```python
from build123d import *

# Parameters (mm, degrees)
SKETCH1_R           = 55
SKETCH1_R_2         = 3
BOSS_EXTRUDE1_DEPTH = 10
CUT_EXTRUDE1_DEPTH  = 10


with BuildPart() as part:
    # Sketch1 → Boss-Extrude1 (new body)
    with BuildSketch(Plane.XY):
        Circle(SKETCH1_R)
        Circle(SKETCH1_R_2, mode=Mode.SUBTRACT)
    extrude(amount=BOSS_EXTRUDE1_DEPTH)

    # Sketch2 → Cut-Extrude1 (cut)
    with BuildSketch(Plane.XY.offset(10)):
        with BuildLine():
            Line((-50.754310162, -5), (-46.733285782, -5))
            ThreePointArc((-46.733285782, -5), (0, -47), (46.733285782, -5))
            Line((46.733285782, -5), (50.754310162, -5))
            ThreePointArc((50.754310162, -5), (0, -51), (-50.754310162, -5))
        make_face()
        with BuildLine():
            Line((-50.754310162, 5), (-46.733285782, 5))
            ThreePointArc((-46.733285782, 5), (0, 47), (46.733285782, 5))
            Line((46.733285782, 5), (50.754310162, 5))
            ThreePointArc((50.754310162, 5), (0, 51), (-50.754310162, 5))
        make_face()
    extrude(amount=-CUT_EXTRUDE1_DEPTH, mode=Mode.SUBTRACT)


solid = part.part
```
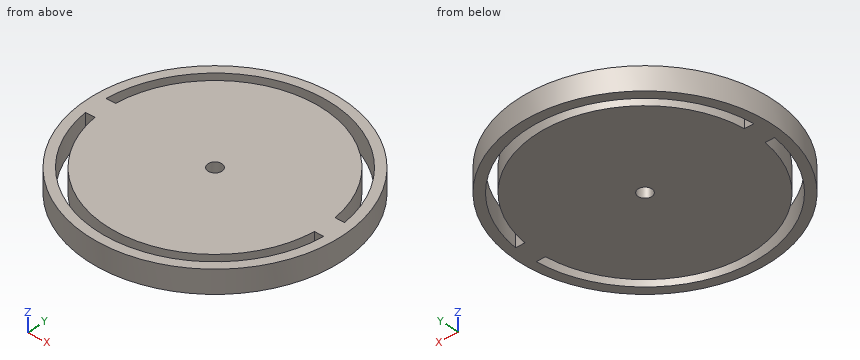
The model under review builds one solid part; all positions refer to its coordinate system, in mm. Coordinates: 2 decimals unless noted, no trailing zeros. Write each loop counter-clockwise with the first axis right and the second up, starting at its lowest first coordinate (ties: lowest second). Pieces come first, ordered by that corner, then holes. Notation, with made-up numbers: (46, -8) - (85, -8) arc R18 ccw to (85, 4) - close; hole circle Ø11 at (-14.75, 63.5). An arc over 180 degrees is marked (long way). Answer in a Markdown table with one row per item. Add a question column.
Q1. Consider section D-D on x = -11. Give the boundary of the cut face in (y, z).
Q2. Consider section B-B on z = 7. Give the boundary of the cut face in (x, y).
Q3. Consider section C-C on x = 0. Give the boundary of the cut face in (y, z).
Q4. Clearance check with flat-ended pins moving along their axes: pin 1 (3 mm diameter, centred on x = -48.5, z = 5, fed in from -Y); pin 2 (7 mm diameter, centred on x = 0, y = 0, fed in from +Z); pin 3 (4.5 mm diameter, centred on x = 49, z = 6.5, fed in from -Y); pin 4 (2 mm diameter, centred on y = -1.5, z = 8, fed in from +X). State where each tip first meets the part, or that it passes through.
Q5. Consider section A-A on y = 0. Give the boundary of the cut face in (x, z).
Q6. To check wall thickness, follow line 1 along Y through (x, z) = (0, 2.75); line 2 along X through (y, z) = (-13, 6.5); line 3 along X through (y, z) = (41, 5.5). State the ranges of each line that lie inside material, in increasing order. Write a range as from..to.
Answers below:
| question | item | result |
|---|---|---|
| 1 | outline | (-53.89, 0) - (-49.8, 0) - (-49.8, 10) - (-53.89, 10) - close; (-45.69, 0) - (45.69, 0) - (45.69, 10) - (-45.69, 10) - close; (49.8, 0) - (53.89, 0) - (53.89, 10) - (49.8, 10) - close |
| 2 | outline | circle Ø110 at (0, 0); hole (-50.75, -5) arc R51 ccw to (50.75, -5) - (46.73, -5) arc R47 cw to (-46.73, -5) - close; hole (-50.75, 5) - (-46.73, 5) arc R47 cw to (46.73, 5) - (50.75, 5) arc R51 ccw to start; hole circle Ø6 at (0, 0) |
| 3 | outline | (-55, 0) - (-51, 0) - (-51, 10) - (-55, 10) - close; (-47, 0) - (-3, 0) - (-3, 10) - (-47, 10) - close; (3, 0) - (47, 0) - (47, 10) - (3, 10) - close; (51, 0) - (55, 0) - (55, 10) - (51, 10) - close |
| 4 | pin 1 | y = -28.57 |
| 4 | pin 2 | z = 10 |
| 4 | pin 3 | y = -28.97 |
| 4 | pin 4 | x = 55 |
| 5 | outline | (-55, 0) - (-3, 0) - (-3, 10) - (-55, 10) - close; (3, 0) - (55, 0) - (55, 10) - (3, 10) - close |
| 6 | line 1 | -55..-51, -47..-3, 3..47, 51..55 |
| 6 | line 2 | -53.44..-49.32, -45.17..45.17, 49.32..53.44 |
| 6 | line 3 | -36.66..-30.33, -22.98..22.98, 30.33..36.66 |
